Can you work these out from the model? Positions are in its coordinate system, mm. A direction names the side the tool comes from. Give positions to 0.01 mm unless a question says otherwise; leave off trailing zeros. Loops run counter-clockwise (first coordinate to the right, second up) from the corner with the lowest first, then second, coordinate; pieces in that order, holes last. Notation, with made-up numbers: (23, 89.5) -> (65, 89.5) arc R28 cw to (65, 128.5) -> close; hole circle Ø5 at (65, -5.75). An arc over 180 degrees is marked (long way). Return JSON: item names as keys, results as strings. Group by question number.
Q1. Will these pins go through, and if not, where does the flat tip stop? pin 1 (2 mm diameter, centred on y = 0, z = 0, fed in from +X); pin 2 (1 mm diameter, centred on x = -5, y = 1.5, fed in from +Z).
Q2. I need wall thicknesses on line 1 along Z through (x, y) = (-4.5, 0); line 2 along Y through (x, z) = (-4.75, 0) (3 decimals); line 3 along Y through (x, z) = (-8, -1) (3 decimals). Which ranges of each line are inside material? Lowest first, please. Write a range as [from, to].
Q3. Thinking about a two-plate mould opening in Z: for faces 3 (the flat face through (-47.625, 1, 1)), 4 (the flat face through (-23.479, -1.61, -2.737)), 5 (the cylindrical face through (-4.494, -1.103, -0.245)), which applies, pulls with the +Z half, pulls with the -Z half, needs draft (parallel to the pull), parting line crosses it, or undercut?
Q4. Which directions (+Z, -Z, +X, -X, +Y, -Y) give clear straight access to the entire face, cutting with the end or side of a thin tool? Please do faces 1 (the flat face through (-23, 3.175, 0)), 2 (the cylindrical face through (-43.131, -1.103, 0.245)).
Q5. Suppose I cut it at A-A, the plane x = -44. Please give me the cut outline in (y, z) (3 decimals), and give its area (3 significant figures).
Q6. Suppose I cut it at C-C, the plane y = -1.75. Please give me the cut outline in (x, z) (3 decimals), and give its area (3 significant figures).
Q7. Suppose I cut it at B-B, the plane x = -18. Please give me the cut outline in (y, z) (3 decimals).
Q8. Suppose I cut it at D-D, the plane z = -3. Please give me the cut outline in (x, y) (3 decimals).
```python
from build123d import *

# Parameters (mm, degrees)
EXTRUDE1_DEPTH            = 47.625
F_4_40_TAPPED_HOLE1_D     = 2.2606
F_4_40_TAPPED_HOLE1_DEPTH = 8.8646
F_4_40_TAPPED_HOLE1_TIP   = 0.679152758
F_4_40_TAPPED_HOLE2_D     = 2.2606
F_4_40_TAPPED_HOLE2_DEPTH = 8.8646
F_4_40_TAPPED_HOLE2_TIP   = 0.679152758


with BuildPart() as part:
    # Sketch1 → Extrude1 (new body)
    with BuildSketch(Plane(origin=(0, 0, 0), x_dir=(0, 0, -1), z_dir=(1, 0, 0))):
        Polygon((3.666174209, 0), (1.833087105, 3.175), (-1.833087105, 3.175), (-3.666174209, 0), (-1.833087105, -3.175), (1.833087105, -3.175), align=None)
    extrude(amount=-EXTRUDE1_DEPTH)

    # #4-40 Tapped Hole1
    with Locations(Plane(origin=(0, 0, 0), x_dir=(0, 0, -1), z_dir=(1, 0, 0))):
        with Locations((0, 0)):
            Hole(F_4_40_TAPPED_HOLE1_D / 2, depth=F_4_40_TAPPED_HOLE1_DEPTH)
            with Locations((0, 0, -(F_4_40_TAPPED_HOLE1_DEPTH + F_4_40_TAPPED_HOLE1_TIP / 2))):  # 118° drill point
                Cone(0, F_4_40_TAPPED_HOLE1_D / 2, F_4_40_TAPPED_HOLE1_TIP, mode=Mode.SUBTRACT)

    # #4-40 Tapped Hole2
    with Locations(Plane.ZY.offset(47.625)):
        with Locations((0, 0)):
            Hole(F_4_40_TAPPED_HOLE2_D / 2, depth=F_4_40_TAPPED_HOLE2_DEPTH)
            with Locations((0, 0, -(F_4_40_TAPPED_HOLE2_DEPTH + F_4_40_TAPPED_HOLE2_TIP / 2))):  # 118° drill point
                Cone(0, F_4_40_TAPPED_HOLE2_D / 2, F_4_40_TAPPED_HOLE2_TIP, mode=Mode.SUBTRACT)


solid = part.part
```
Ans:
{
 "1": {"pin 1": "stops at x = -8.94", "pin 2": "stops at z = 3.09"},
 "2": {"line 1": "z = [-3.67, -1.13], [1.13, 3.67]", "line 2": "y = [-3.175, -1.13], [1.13, 3.175]", "line 3": "y = [-3.175, -0.527], [0.527, 3.175]"},
 "3": {"face 3": "needs draft", "face 4": "pulls with the -Z half", "face 5": "undercut"},
 "4": {"face 1": "+Z, -Z, +X, -X, +Y", "face 2": "-X"},
 "5": {"outline": "(-3.175, -1.833) -> (0, -3.666) -> (3.175, -1.833) -> (3.175, 1.833) -> (0, 3.666) -> (-3.175, 1.833) -> close; hole circle Ø2.261 at (0, 0)", "area": "30.9 mm^2"},
 "6": {"outline": "(-47.625, -2.656) -> (0, -2.656) -> (0, 2.656) -> (-47.625, 2.656) -> close", "area": "253 mm^2"},
 "7": {"outline": "(-3.175, -1.833) -> (0, -3.666) -> (3.175, -1.833) -> (3.175, 1.833) -> (0, 3.666) -> (-3.175, 1.833) -> close"},
 "8": {"outline": "(-47.625, -1.154) -> (0, -1.154) -> (0, 1.154) -> (-47.625, 1.154) -> close"}
}
